Part model, mm, in its own coordinate system. A direction names the side the tool comes from. Give positions to 0.01 mm unless a question says otherwise; leave off trailing zeros. Order: outer loops, then holes, each group sorted by start corner. A loop starts at its lowest first (then second) coordinate and runs counter-clockwise, first axis right, second up. Notation, with made-up numbers: M 83.25,23.25 L 102.25,23.25 A33 ccw 102.25,60.25 Z; hole C -34,45.5 d10. An arc over 180 degrees is marked long. Return JSON: item names as keys, results as strings.
from build123d import *

# Parameters (mm, degrees)
SKETCH_1_W                      = 110
SKETCH_1_H                      = 70
EXTRUDE_1_DEPTH                 = 5
EXTRUDE_2_DEPTH                 = 70
CUT_EXTRUDE_2_DEPTH             = 70
EXTRUDE_3_DEPTH                 = 20
SKETCH_5_R                      = 1.5
CUT_EXTRUDE_3_DEPTH             = 10
SKETCH_6_R                      = 1.5
CUT_EXTRUDE_4_DEPTH             = 10
CUT_EXTRUDE_5_REACH             = 145.602
SKETCH_7_R                      = 1.5
CUT_EXTRUDE_5_DIRECTION_2_DEPTH = 144.601807274
SKETCH_8_R                      = 3
CUT_EXTRUDE_6_DEPTH             = 3
CUT_EXTRUDE_7_REACH             = 145.602
SKETCH_9_R                      = 1
FILLET_1_R                      = 4
SKETCH_10_R                     = 1.5
CUT_EXTRUDE_8_DEPTH             = 10


with BuildPart() as part:
    # 草图1 → 凸台-拉伸1 (new body)
    with BuildSketch(Plane(origin=(0, 0, 0), x_dir=(1, 0, 0), z_dir=(0, 1, 0))):
        with Locations((55, 35)):
            Rectangle(SKETCH_1_W, SKETCH_1_H)
    extrude(amount=EXTRUDE_1_DEPTH)

    # 草图2 → 凸台-拉伸2 (add)
    with BuildSketch(Plane(origin=(0, 0, -70), x_dir=(-1, 0, 0), z_dir=(0, 0, -1))):
        with BuildLine():
            Line((0, 0), (-110, 0))
            Line((-110, 0), (-110, -8.38034143))
            ThreePointArc((-110, -8.38034143), (-101.497088177, -9.012210946), (-96.000017961, -15.529955003))
            Line((-96.000017961, -15.529955003), (-94.999994392, -15.529955003))
            ThreePointArc((-94.999994392, -15.529955003), (-84.5, -7.808692226), (-74.000005608, -15.529955003))
            Line((-74.000005608, -15.529955003), (-72.999994392, -15.529955003))
            ThreePointArc((-72.999994392, -15.529955003), (-62.5, -7.808692226), (-52.000005608, -15.529955003))
            Line((-52.000005608, -15.529955003), (-50.999994392, -15.529955003))
            ThreePointArc((-50.999994392, -15.529955003), (-40.5, -7.808692226), (-30.000005608, -15.529955003))
            Line((-30.000005608, -15.529955003), (-29.000017961, -15.529955003))
            ThreePointArc((-29.000017961, -15.529955003), (-25.01669227, -9.946792076), (-18.500017961, -7.808674266))
            Line((-18.500017961, -7.808674266), (0, -7.808674266))
            Line((0, -7.808674266), (0, 0))
        make_face()
    extrude(amount=-EXTRUDE_2_DEPTH)

    # 草图3 → 切除-拉伸2 (cut)
    with BuildSketch(Plane(origin=(0, 0, -70), x_dir=(-1, 0, 0), z_dir=(0, 0, -1))):
        with BuildLine():
            Line((-96.000017961, -15.529955003), (-95.790676244, -15.529955003))
            ThreePointArc((-95.790676244, -15.529955003), (-101.348565543, -8.863698751), (-110, -8.169589449))
            Line((-110, -8.169589449), (-110, -8.38034143))
            ThreePointArc((-110, -8.38034143), (-101.497088177, -9.012210946), (-96.000017961, -15.529955003))
        make_face()
        with BuildLine():
            ThreePointArc((-73.790676244, -15.529955003), (-84.500017961, -7.608674266), (-95.209359677, -15.529955003))
            Line((-95.209359677, -15.529955003), (-94.999994392, -15.529955003))
            ThreePointArc((-94.999994392, -15.529955003), (-84.5, -7.808692226), (-74.000005608, -15.529955003))
            Line((-74.000005608, -15.529955003), (-73.790676244, -15.529955003))
        make_face()
        with BuildLine():
            ThreePointArc((-51.790676244, -15.529955003), (-62.500017961, -7.608674266), (-73.209359677, -15.529955003))
            Line((-73.209359677, -15.529955003), (-72.999994392, -15.529955003))
            ThreePointArc((-72.999994392, -15.529955003), (-62.5, -7.808692226), (-52.000005608, -15.529955003))
            Line((-52.000005608, -15.529955003), (-51.790676244, -15.529955003))
        make_face()
        with BuildLine():
            ThreePointArc((-29.790676244, -15.529955003), (-40.500017961, -7.608674266), (-51.209359677, -15.529955003))
            Line((-51.209359677, -15.529955003), (-50.999994392, -15.529955003))
            ThreePointArc((-50.999994392, -15.529955003), (-40.5, -7.808692226), (-30.000005608, -15.529955003))
            Line((-30.000005608, -15.529955003), (-29.790676244, -15.529955003))
        make_face()
        with BuildLine():
            Line((-18.500017961, -7.808674266), (-16.39288721, -7.808674266))
            ThreePointArc((-16.39288721, -7.808674266), (-24.279641861, -9.215137505), (-29.209359677, -15.529955003))
            Line((-29.209359677, -15.529955003), (-29.000017961, -15.529955003))
            ThreePointArc((-29.000017961, -15.529955003), (-25.01669227, -9.946792076), (-18.500017961, -7.808674266))
        make_face()
    extrude(amount=-CUT_EXTRUDE_2_DEPTH, mode=Mode.SUBTRACT)

    # 草图4 → 凸台-拉伸3 (add)
    with BuildSketch(Plane(origin=(0, 0, -70), x_dir=(-1, 0, 0), z_dir=(0, 0, -1))):
        Polygon((0, 5), (-110, 5), (-110, -7.608674266), (-7.3, -7.608674266), (-7.3, -7.808674266), (0, -7.808674266), (0, -7.608674266), align=None)
    extrude(amount=EXTRUDE_3_DEPTH)

    # 草图5 → 切除-拉伸3 (cut)
    with BuildSketch(Plane.XY):
        with Locations((95.50000898, -1)):
            Circle(SKETCH_5_R)
        with Locations((29.49999102, -1)):
            Circle(SKETCH_5_R)
    extrude(amount=-CUT_EXTRUDE_3_DEPTH, mode=Mode.SUBTRACT)

    # 草图6 → 切除-拉伸4 (cut)
    with BuildSketch(Plane(origin=(110, 0, 0), x_dir=(0, 0, -1), z_dir=(1, 0, 0))):
        with Locations((78, -1.304337133)):
            Circle(SKETCH_6_R)
        with Locations((12, -1.304337133)):
            Circle(SKETCH_6_R)
    extrude(amount=-CUT_EXTRUDE_4_DEPTH, mode=Mode.SUBTRACT)

    # 草图7 → 切除-拉伸5 (cut, up to next)
    with BuildSketch(Plane(origin=(0, 5, 0), x_dir=(1, 0, 0), z_dir=(0, 1, 0)), mode=Mode.PRIVATE) as cut_extrude_5_sk1:
        with Locations(Location((3.65000898, 78, 0), (0, 0, 90))):
            Circle(SKETCH_7_R)
    cut_extrude_5_tool1 = extrude(cut_extrude_5_sk1.sketch, amount=-CUT_EXTRUDE_5_REACH, mode=Mode.PRIVATE) & part.part
    # 草图7 → 切除-拉伸5 (cut, up to next)
    with BuildSketch(Plane(origin=(0, 5, 0), x_dir=(1, 0, 0), z_dir=(0, 1, 0)), mode=Mode.PRIVATE) as cut_extrude_5_sk2:
        with Locations(Location((3.65000898, 12, 0), (0, 0, 90))):
            Circle(SKETCH_7_R)
    cut_extrude_5_tool2 = extrude(cut_extrude_5_sk2.sketch, amount=-CUT_EXTRUDE_5_REACH, mode=Mode.PRIVATE) & part.part
    add(cut_extrude_5_tool1.solids().sort_by_distance((3.650009, 5, -78))[0], mode=Mode.SUBTRACT)
    add(cut_extrude_5_tool2.solids().sort_by_distance((3.650009, 5, -12))[0], mode=Mode.SUBTRACT)

    # 草图7 → 切除-拉伸5 direction 2 (cut)
    with BuildSketch(Plane(origin=(0, 5, 0), x_dir=(1, 0, 0), z_dir=(0, 1, 0))):
        with Locations(Location((3.65000898, 78, 0), (0, 0, 90))):
            Circle(SKETCH_7_R)
        with Locations(Location((3.65000898, 12, 0), (0, 0, 90))):
            Circle(SKETCH_7_R)
    extrude(amount=CUT_EXTRUDE_5_DIRECTION_2_DEPTH, mode=Mode.SUBTRACT)

    # 草图8 → 切除-拉伸6 (cut)
    with BuildSketch(Plane(origin=(0, 5, 0), x_dir=(1, 0, 0), z_dir=(0, 1, 0))):
        with Locations(Location((3.65000898, 12, 0), (0, 0, 270))):
            Circle(SKETCH_8_R)
        with Locations(Location((3.65000898, 78, 0), (0, 0, 270))):
            Circle(SKETCH_8_R)
    extrude(amount=-CUT_EXTRUDE_6_DEPTH, mode=Mode.SUBTRACT)

    # 草图9 → 切除-拉伸7 (cut, up to next)
    with BuildSketch(Plane(origin=(0, 5, 0), x_dir=(1, 0, 0), z_dir=(0, 1, 0)), mode=Mode.PRIVATE) as cut_extrude_7_sk1:
        with Locations(Location((14.442, 62.109, 0), (0, 0, 270))):
            Circle(SKETCH_9_R)
    cut_extrude_7_tool1 = extrude(cut_extrude_7_sk1.sketch, amount=-CUT_EXTRUDE_7_REACH, mode=Mode.PRIVATE) & part.part
    add(cut_extrude_7_tool1.solids().sort_by_distance((14.442, 5, -62.109))[0], mode=Mode.SUBTRACT)

    # 圆角1
    # the kernel refuses this fillet: 4 mm, written as the material it takes off along each edge
    with BuildSketch(Plane(origin=(0, 5, 10), x_dir=(0, -1, 0), z_dir=(0, 0, -1))) as fillet_1_piece_1:
        with BuildLine():
            CenterArc((FILLET_1_R, -FILLET_1_R), FILLET_1_R, 90, 90)
            Line((0, -FILLET_1_R), (0, 0))
            Line((0, 0), (FILLET_1_R, 0))
        make_face()
    extrude(amount=110, mode=Mode.SUBTRACT)

    # 草图10 → 切除-拉伸8 (cut)
    with BuildSketch(Plane(origin=(0, 0, -90), x_dir=(-1, 0, 0), z_dir=(0, 0, -1))):
        with Locations((-62.5, -1.304337133)):
            Circle(SKETCH_10_R)
    extrude(amount=-CUT_EXTRUDE_8_DEPTH, mode=Mode.SUBTRACT)


solid = part.part
Q1. Probe line 1 along X through (y, z) = (-3.75, -12); line 2 along X through (y, z) = (-13, -19); line 3 along X through (y, z) = (-10.5, -30). List the from-to ranges inside material, lowest first.
Established:
{"line 1": "x = 0 to 2.15, 5.15 to 110", "line 2": "x = 28.08 to 30.92, 50.08 to 52.92, 72.08 to 74.92, 94.08 to 96.92", "line 3": "x = 26.01 to 32.99, 48.01 to 54.99, 70.01 to 76.99, 92.01 to 98.99"}
Q2. Band-saw the part on A-A (z = -7.5). Give the cut face in (x, y).
Established:
{"outline": "M 0,-7.81 L 16.39,-7.81 A11.2 cw 29.21,-15.53 L 29.79,-15.53 A11.2 cw 51.21,-15.53 L 51.79,-15.53 A11.2 cw 73.21,-15.53 L 73.79,-15.53 A11.2 cw 95.21,-15.53 L 95.79,-15.53 A11.2 cw 110,-8.17 L 110,5 L 4,5 A4 ccw 0,1 Z; hole C 29.5,-1 d3; hole C 95.5,-1 d3"}
Q3. Band-saw the part on C-C (y = -14). Give the cut face in (x, z), then the cut area to 3 significant figures.
Established:
{"outline": "M 28.62,-70 L 30.38,-70 L 30.38,0 L 28.62,0 Z; M 50.62,-70 L 52.38,-70 L 52.38,0 L 50.62,0 Z; M 72.62,-70 L 74.38,-70 L 74.38,0 L 72.62,0 Z; M 94.62,-70 L 96.38,-70 L 96.38,0 L 94.62,0 Z", "area": "496 mm²"}
Q4. Band-saw the part on D-D (x = 22.5). Give the cut face in (y, z).
Established:
{"outline": "M -8.35,-70 L -7.61,-70 L -7.61,-90 L 5,-90 L 5,0 L -8.35,0 Z"}
Q5. Band-saw the part on B-B (z = -46.5). Give the cut face in (x, y).
Established:
{"outline": "M 0,-7.81 L 16.39,-7.81 A11.2 cw 29.21,-15.53 L 29.79,-15.53 A11.2 cw 51.21,-15.53 L 51.79,-15.53 A11.2 cw 73.21,-15.53 L 73.79,-15.53 A11.2 cw 95.21,-15.53 L 95.79,-15.53 A11.2 cw 110,-8.17 L 110,5 L 4,5 A4 ccw 0,1 Z"}
Q6. 3-axis set-ups, long thin cutter, end or side, ignore diameter. For faces 1 (the flat face through (30, -10, -70)), 2 (the flat face through (100, -1, -78)), 3 (the flat face through (5, 2, -11)): which of +Z, -Z, +X, -X, +Y, -Y reach the whole face in a straight line?
Established:
{"face 1": "-Z, +X, -Y", "face 2": "+X", "face 3": "+Y"}
Q7. Two-plate mould, pull along Y, no slides. Class faces 4 (the cylindrical face through (105.07, -2.22, -10.81)), 5 (the flat face through (0, -3, -44)), 6 (the flat face through (59, -7.609, -80)), 7 (the cylindrical face through (1.141, 3.797, -44.37)): +Y half, -Y half, draft (parallel to the pull), parting line (faces both ways), or undercut.
Established:
{"face 4": "undercut", "face 5": "draft", "face 6": "-Y half", "face 7": "+Y half"}
Q8. Pin check, flat tips, straight feed: pin 1 (1.8 mm diameter, centred on x = 14.442, z = -62.109, fed in from -Y); pin 2 (10 mm diameter, centred on x = 67, z = -81.5, fed in from -Y); pin 3 (2 mm diameter, centred on x = 36.5, z = -37, fed in from -Y); pin 4 (1.5 mm diameter, centred on y = 3, z = -74, fed in from -X). Stop position of each tip, or through.
Established:
{"pin 1": "passes through", "pin 2": "stops at y = -7.61", "pin 3": "stops at y = -8.79", "pin 4": "stops at x = 0.2"}
